from build123d import *

# Parameters (mm, degrees)
F0_W     = 175.97738
F0_H     = 127.75816
F1_DEPTH = 25.4
F2_R     = 33.3375
F3_DEPTH = 25.4
F4_R     = 26.559613
F5_DEPTH = 25.4


with BuildPart() as f1:
    # F0 (on Front) → F1 (new body)
    with BuildSketch(Plane.XZ):
        Rectangle(F0_W, F0_H)
    extrude(amount=F1_DEPTH)

    # F2 (on face) → F3 (intersect)
    with BuildSketch(Plane.XZ.offset(25.4)):
        Circle(F2_R)
    extrude(amount=-F3_DEPTH, mode=Mode.INTERSECT)

    # F4 (on face) → F5 (cut)
    with BuildSketch(Plane.XZ.offset(25.4)):
        Circle(F4_R)
    extrude(amount=-F5_DEPTH, mode=Mode.SUBTRACT)


solid = f1.part
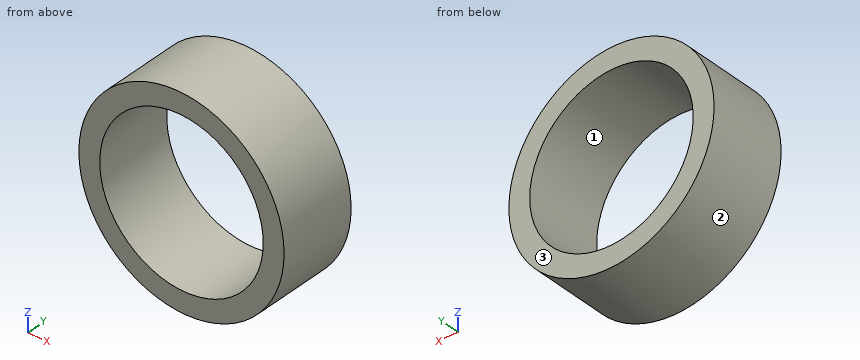
The listing builds one solid part. Answer for the finished solid, in the listing's coordinates (mm). Face numbers are marked on the shaded views. Coordinates: 2 decimals unless noted, no trailing zeros. Loops run counter-clockwise (first coordinate to the right, second up) from the corner with the lowest first, then second, coordinate; pieces in that order, holes last.
1) Flat-ended cylindrical pins translate along their axes: pin 1 Ø5 at (y, z) = (-2.5, 16) entering from +X; pin 2 Ø12 at (x, y) = (-23.5, -20.5) entering from +Z; pin 3 Ø3 at (x, y) = (16.5, -21.5) entering from -Z. Find the tip coordinate at first contact, or state that the pin passes through.
2) Find section B-B on z = 0. Write down the section's boundary in (x, y), then the cut area to 3 significant figures.
3) Determine the mould class of the marked faces 1, 2 and 3 for opening direction X: pulls with the +X half, pulls with the -X half, needs draft (parallel to the pull), parting line crosses it, or undercut.
4) Find section A-A on x = 0. Write down the section's boundary in (y, z).
5) Find section C-C on y = -18.75. Write down the section's boundary in (x, z) (1 decimal), then the cut area to 3 significant figures.
6) Find the intervals of material crossed by L1, parallel to Z at x = 0, y = -7.5; L2, parallel to X at y = -2, z = -15.5; L3, parallel to Z at x = 2, y = -21, in increasing order.
Values:
1. pin 1: stops at x = 30.48
1. pin 2: stops at z = 28.37
1. pin 3: stops at z = -29.77
2. outline: (-33.34, -25.4) - (-26.56, -25.4) - (-26.56, 0) - (-33.34, 0) - close; (26.56, -25.4) - (33.34, -25.4) - (33.34, 0) - (26.56, 0) - close
2. area: 344 mm2
3. face 1: undercut
3. face 2: parting line crosses it
3. face 3: needs draft
4. outline: (-25.4, -33.34) - (0, -33.34) - (0, -26.56) - (-25.4, -26.56) - close; (-25.4, 26.56) - (0, 26.56) - (0, 33.34) - (-25.4, 33.34) - close
5. outline: circle Ø66.7 at (0, 0); hole circle Ø53.1 at (0, 0)
5. area: 1,280 mm2
6. L1: z = -33.34 to -26.56, 26.56 to 33.34
6. L2: x = -29.52 to -21.57, 21.57 to 29.52
6. L3: z = -33.28 to -26.48, 26.48 to 33.28
